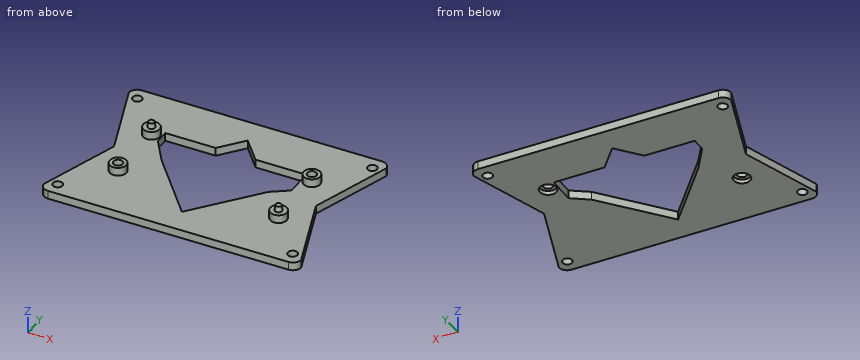
from build123d import *
from OCP.BRepFilletAPI import BRepFilletAPI_MakeChamfer

# Parameters (mm, degrees)
SKETCH2_W           = 93
SKETCH2_H           = 64.518072289
SKETCH2_R           = 1.740963855
BOSS_EXTRUDE1_DEPTH = 3
FILLET1_R           = 3
SKETCH3_R           = 3
SKETCH3_R_2         = 1.325
BOSS_EXTRUDE2_DEPTH = 3
SKETCH4_R           = 1.3
BOSS_EXTRUDE3_DEPTH = 2
SKETCH5_R           = 1.7
CUT_EXTRUDE1_DEPTH  = 11
CHAMFER1_SIZE       = 2
CHAMFER1_SIZE_2     = 0.25
CUT_EXTRUDE2_DEPTH  = 11
CUT_EXTRUDE3_DEPTH  = 11
SKETCH8_R           = 3
SKETCH8_R_2         = 1.7
CUT_EXTRUDE4_DEPTH  = 1.5
CUT_EXTRUDE5_DEPTH  = 1.5
CUT_EXTRUDE6_DEPTH  = 3


with BuildPart() as part:
    # Sketch2 → Boss-Extrude1 (new body)
    with BuildSketch(Plane.XY):
        with Locations((46.5, 32.259036145)):
            Rectangle(SKETCH2_W, SKETCH2_H)
        with Locations((89, 4.759036145)):
            Circle(SKETCH2_R, mode=Mode.SUBTRACT)
        with Locations((89, 59.759036145)):
            Circle(SKETCH2_R, mode=Mode.SUBTRACT)
        with Locations((4, 59.759036145)):
            Circle(SKETCH2_R, mode=Mode.SUBTRACT)
        with Locations((4, 4.759036145)):
            Circle(SKETCH2_R, mode=Mode.SUBTRACT)
    extrude(amount=BOSS_EXTRUDE1_DEPTH)

    # Fillet1
    fillet1_edges = [part.edges().sort_by_distance(p)[0] for p in [
        (0, 0, 1.5),
        (0, 64.518072289, 1.5),
        (93, 64.518072289, 1.5),
        (93, 0, 1.5),
    ]]
    fillet(fillet1_edges, radius=FILLET1_R)

    # Sketch3 → Boss-Extrude2 (add)
    # profile 1 of 8: a face of its own
    with BuildSketch(Plane.XY.offset(3)):
        with Locations((17.475, 43.784036145)):
            Circle(SKETCH3_R)
        with Locations((17.475, 43.784036145)):
            Circle(SKETCH3_R_2, mode=Mode.SUBTRACT)
    # profile 2 of 8: a face of its own
    with BuildSketch(Plane.XY.offset(3)):
        with Locations((17.475, 20.734036145)):
            Circle(SKETCH3_R)
        with Locations((17.475, 20.734036145)):
            Circle(SKETCH3_R_2, mode=Mode.SUBTRACT)
    # profile 3 of 8: a face of its own
    with BuildSketch(Plane.XY.offset(3)):
        with Locations((17.475, 20.734036145)):
            Circle(SKETCH3_R_2)
    # profile 4 of 8: a face of its own
    with BuildSketch(Plane.XY.offset(3)):
        with Locations((75.525, 43.784036145)):
            Circle(SKETCH3_R)
        with Locations((75.525, 43.784036145)):
            Circle(SKETCH3_R_2, mode=Mode.SUBTRACT)
    # profile 5 of 8: a face of its own
    with BuildSketch(Plane.XY.offset(3)):
        with Locations((75.525, 43.784036145)):
            Circle(SKETCH3_R_2)
    # profile 6 of 8: a face of its own
    with BuildSketch(Plane.XY.offset(3)):
        with Locations((75.525, 20.734036145)):
            Circle(SKETCH3_R)
        with Locations((75.525, 20.734036145)):
            Circle(SKETCH3_R_2, mode=Mode.SUBTRACT)
    # profile 7 of 8: a face of its own
    with BuildSketch(Plane.XY.offset(3)):
        with Locations((75.525, 20.734036145)):
            Circle(SKETCH3_R_2)
    # profile 8 of 8: a face of its own
    with BuildSketch(Plane.XY.offset(3)):
        with Locations((17.475, 43.784036145)):
            Circle(SKETCH3_R_2)
    extrude(amount=BOSS_EXTRUDE2_DEPTH)

    # Sketch4 → Boss-Extrude3 (add)
    with BuildSketch(Plane.XY.offset(6)):
        with Locations((75.525, 20.734036145)):
            Circle(SKETCH4_R)
        with Locations((17.475, 43.784036145)):
            Circle(SKETCH4_R)
    extrude(amount=BOSS_EXTRUDE3_DEPTH)

    # Sketch5 → Cut-Extrude1 (cut)
    with BuildSketch(Plane.XY.offset(6)):
        with Locations((17.475, 20.734036145)):
            Circle(SKETCH5_R)
        with Locations((75.525, 43.784036145)):
            Circle(SKETCH5_R)
    extrude(amount=-CUT_EXTRUDE1_DEPTH, mode=Mode.SUBTRACT)

    # Chamfer1
    chamfer1_edges_1 = [part.edges().sort_by_distance(p)[0] for p in [
        (74.225, 20.734036145, 8),
    ]]
    chamfer1_side_1 = [part.faces().sort_by_distance(p)[0] for p in [
        (74.225, 20.734036145, 7.995),
    ]]
    chamfer1_edges_2 = [part.edges().sort_by_distance(p)[0] for p in [
        (16.175, 43.784036145, 8),
    ]]
    chamfer1_side_2 = [part.faces().sort_by_distance(p)[0] for p in [
        (16.175, 43.784036145, 7.995),
    ]]
    chamfer1 = BRepFilletAPI_MakeChamfer(part.part.solid().wrapped)
    for e in chamfer1_edges_1:
        chamfer1.Add(CHAMFER1_SIZE - 0.0001, CHAMFER1_SIZE_2 - 0.0001, e.wrapped, chamfer1_side_1[0].wrapped)
    for e in chamfer1_edges_2:
        chamfer1.Add(CHAMFER1_SIZE - 0.0001, CHAMFER1_SIZE_2 - 0.0001, e.wrapped, chamfer1_side_2[0].wrapped)
    add(Compound.cast(chamfer1.Shape()), mode=Mode.REPLACE)  # a hair under: the kernel refuses the full size

    # Sketch6 → Cut-Extrude2 (cut)
    with BuildSketch(Plane.XY.offset(3)):
        Polygon((46.41475966, 55.04295344), (27.196400626, 32.259036144), (46.5, 9.374063974), (65.803599374, 32.259036145), align=None)
    extrude(amount=-CUT_EXTRUDE2_DEPTH, mode=Mode.SUBTRACT)

    # Sketch7 → Cut-Extrude3 (cut)
    with BuildSketch(Plane.XY.offset(3)):
        Polygon((21, 46.559036145), (21, 41.459036145), (66.9, 41.459036145), (66.9, 36.459036145), (72, 36.459036145), (72, 46.559036145), align=None)
    extrude(amount=-CUT_EXTRUDE3_DEPTH, mode=Mode.SUBTRACT)

    # Sketch8 → Cut-Extrude4 (cut)
    # profile 1 of 4: a face of its own
    with BuildSketch(Plane(origin=(0, 0, 0), x_dir=(-1, 0, 0), z_dir=(0, 0, -1))):
        with Locations(Location((-75.525, 43.784036145, 0), (0, 0, 180))):
            Circle(SKETCH8_R)
        with Locations(Location((-75.525, 43.784036145, 0), (0, 0, 180))):
            Circle(SKETCH8_R_2, mode=Mode.SUBTRACT)
    # profile 2 of 4: a face of its own
    with BuildSketch(Plane(origin=(0, 0, 0), x_dir=(-1, 0, 0), z_dir=(0, 0, -1))):
        with Locations(Location((-17.475, 20.734036145, 0), (0, 0, 180))):
            Circle(SKETCH8_R)
        with Locations(Location((-17.475, 20.734036145, 0), (0, 0, 180))):
            Circle(SKETCH8_R_2, mode=Mode.SUBTRACT)
    # profile 3 of 4: a face of its own
    with BuildSketch(Plane(origin=(0, 0, 0), x_dir=(-1, 0, 0), z_dir=(0, 0, -1))):
        Polygon((-72, 36.459036145), (-65.803599374, 32.259036145), (-57.974509975, 41.459036145), (-66.9, 41.459036145), align=None)
    # profile 4 of 4: a face of its own
    with BuildSketch(Plane(origin=(0, 0, 0), x_dir=(-1, 0, 0), z_dir=(0, 0, -1))):
        Polygon((-27.196400626, 32.259036144), (-21, 41.459036145), (-34.956651017, 41.459036145), align=None)
    extrude(amount=-CUT_EXTRUDE4_DEPTH, mode=Mode.SUBTRACT)

    # Sketch9 → Cut-Extrude5 (cut)
    with BuildSketch(Plane(origin=(0, 0, 1.5), x_dir=(-1, 0, 0), z_dir=(0, 0, -1))):
        Polygon((-66.9, 36.459036145), (-72, 36.459036145), (-65.803599374, 32.259036145), (-57.974509975, 41.459036145), (-66.9, 41.459036145), align=None)
        Polygon((-34.956651017, 41.459036145), (-27.196400626, 32.259036144), (-21, 41.459036145), align=None)
    extrude(amount=-CUT_EXTRUDE5_DEPTH, mode=Mode.SUBTRACT)

    # Sketch10 → Cut-Extrude6 (cut)
    with BuildSketch(Plane.XY.offset(3)):
        Polygon((0, 61.518072289), (0, 32.259036145), (10, 32.259036145), align=None)
        Polygon((10, 32.259036145), (0, 32.259036145), (0, 3), align=None)
        Polygon((93, 32.259036145), (93, 61.518072289), (83, 32.259036145), align=None)
        Polygon((83, 32.259036145), (93, 3), (93, 32.259036145), align=None)
    extrude(amount=-CUT_EXTRUDE6_DEPTH, mode=Mode.SUBTRACT)


solid = part.part
Build history of the part. All positions in model axes, mm. Round coordinates to 2 decimals unless told otherwise and drop trailing zeros. Loops run counter-clockwise (first coordinate to the right, second up) from the corner with the lowest first, then second, coordinate; pieces in that order, holes last. Notation, with made-up numbers: (41, 85.5) -> (56, 85.5) arc R9 ccw to (56, 92.5) -> close; hole circle Ø7 at (-23.75, 63.5). An arc over 180 degrees is marked (long way). Use CSV: the item, a comma, the result in double quotes. Start each with the question number.
Q1. Saw through at D-D on x = 89. Give the cut face in (y, z), and give its area (3 significant figures).
Q2. Drill centre lines: L1, parallel to X at y = 58.5, z = 1; L2, parallel to X at y = 41, z = 1.75; L3, parallel to Z at x = 17, y = 13. Where is each one in solid material? Low to high.
Q3. Saw through at C-C on z = 5. Give the cut face in (x, y) (3 decimals), and give its area (3 significant figures).
Q4. Saw through at B-B on x = 8. Give the cut face in (y, z), and give its area (3 significant figures).
Q5. Flat gauge pins, fed straight in: pin 1 Ø3 at (y, z) = (39.5, 1) entering from -X; pin 2 Ø2.5 at (y, z) = (44, 1) entering from -X; pin 3 Ø5 at (x, y) = (18.5, 19.5) entering from +Z. Where does each tip first touch, or does it go through?
Q6. Saw through at A-A on y = 31. Give the cut face in (x, z).
Solutions:
1,outline,"(0, 0) -> (3.02, 0) -> (3.02, 3) -> (0, 3) -> close; (6.5, 0) -> (14.7, 0) -> (14.7, 3) -> (6.5, 3) -> close; (49.81, 0) -> (58.02, 0) -> (58.02, 3) -> (49.81, 3) -> close; (61.5, 0) -> (64.52, 0) -> (64.52, 3) -> (61.5, 3) -> close"
1,area,"67.3 mm^2"
2,L1,"x = 1.03 to 2.8, 5.2 to 87.8, 90.2 to 91.97"
2,L2,"x = 7.01 to 21.31, 72 to 85.99"
2,L3,"z = 0 to 3"
3,outline,"circle Ø6 at (17.475, 20.734); circle Ø6 at (17.475, 43.784); circle Ø6 at (75.525, 20.734); circle Ø6 at (75.525, 43.784); hole circle Ø3.4 at (17.475, 20.734); hole circle Ø3.4 at (75.525, 43.784)"
3,area,"94.9 mm^2"
4,outline,"(0, 0) -> (26.41, 0) -> (26.41, 3) -> (0, 3) -> close; (38.11, 0) -> (64.52, 0) -> (64.52, 3) -> (38.11, 3) -> close"
4,area,"158 mm^2"
5,pin 1,"stops at x = 7.01"
5,pin 2,"stops at x = 5.56"
5,pin 3,"stops at z = 6"
6,outline,"(9.57, 0) -> (28.26, 0) -> (28.26, 3) -> (9.57, 3) -> close; (64.74, 0) -> (83.43, 0) -> (83.43, 3) -> (64.74, 3) -> close"
